For this review, use the dimensioned drawing (mm, ordinates from the lowest corner) and the shaded views. A direction names the side the tool comes from. Coordinates: 2 decimals unless noted, no trailing zeros. Loops run counter-clockwise (first coordinate to the right, second up) from the corner with the lowest first, then second, coordinate; pieces in that order, holes last. Notation, with made-up numbers: (55, 47) - (86, 47) arc R33 cw to (86, 84) - close; hole circle Ø2 at (10.25, 88). An arc over 180 degrees is marked (long way). One line per item, written item: value. Start each with the question number.
1. For the marked faces 5, 6, 7 and 8, list the 3-axis set-ups (+Z, -Z, +X, -X, +Y, -Y) from which the entire face can be reached by the end or side of a thin tool; tool diameter is ignored.
2. To check wall thickness, follow line 1 (Z direction, x = 27.5, y = 14.75); line 2 (Y direction, x = 1.75, z = 13). State the ranges of each line that lie inside material, in increasing order.
3. Insertion check: P1, Ø2.5, axis at y = 2, z = 18.5, coming from the -X side; P2, Ø2, axis at x = 22.5, y = 22, coming from the -Z side; P3, Ø2.5, axis at x = 16.5, z = 2.5, coming from the +Y side. Each pin has a flat end and moves straight along its axis. Give the tip position at first contact, or say it passes through.
4. Mouldability with a two-part tool opening along Z and no side actions: class the marked faces 1, 2, 3 and 4 as +Z half, -Z half, draft (parallel to the pull), parting line (faces both ways), or undercut.
5. We need section C-C, the plane x = 18. Give the boundary of the cut face in (y, z), then the cut area to 3 significant figures.
6. We need section B-B, the plane y = 28. Give the boundary of the cut face in (x, z), then the cut area to 3 significant figures.
7. We need section D-D, the plane x = 26.75. Give the boundary of the cut face in (y, z), then the cut area to 3 significant figures.
8. We need section A-A, the plane z = 23. Give the boundary of the cut face in (x, y).
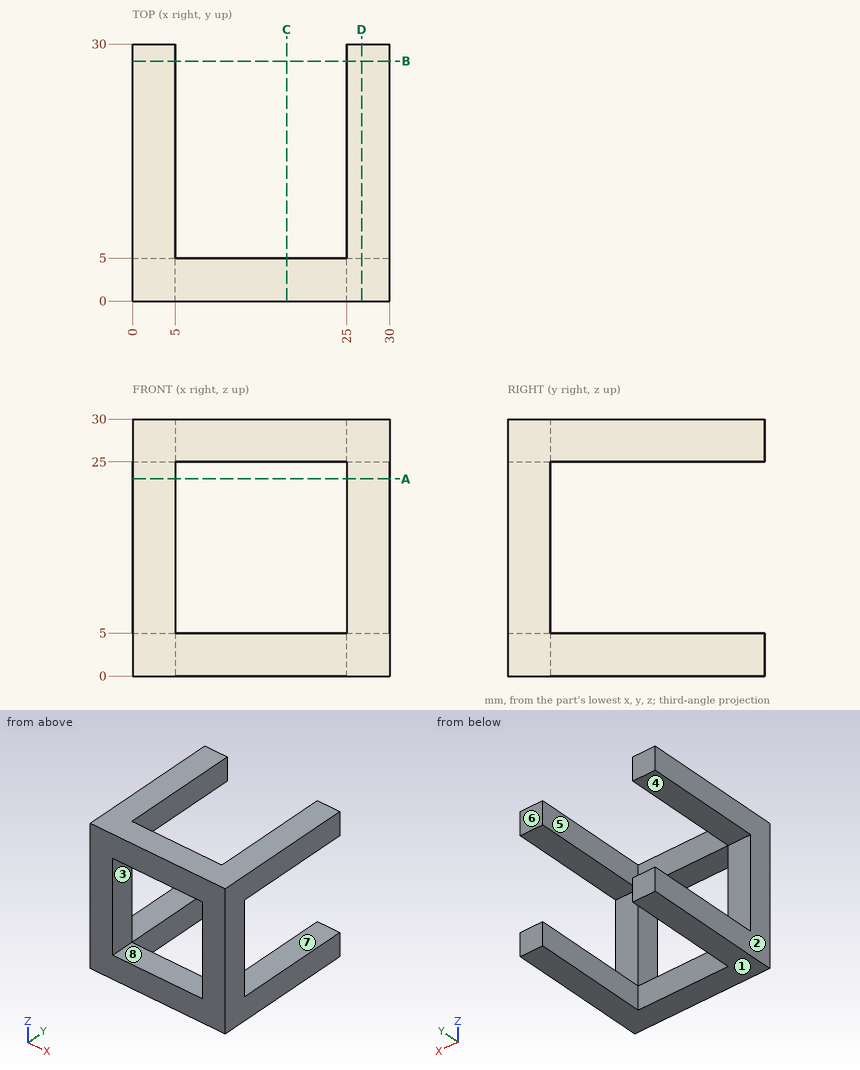
Findings below:
1. face 5: +Z, -Z, +Y
1. face 6: +Z, -Z, +X, -X, +Y
1. face 7: +X, -X, +Y
1. face 8: +Y, -Y
2. line 1: 0 to 5, 25 to 30
2. line 2: 0 to 5
3. P1: x = 0
3. P2: through
3. P3: y = 5
4. face 1: -Z half
4. face 2: draft
4. face 3: undercut
4. face 4: undercut
5. outline: (0, 0) - (5, 0) - (5, 5) - (0, 5) - close; (0, 25) - (5, 25) - (5, 30) - (0, 30) - close
5. area: 50.0 mm2
6. outline: (0, 0) - (5, 0) - (5, 5) - (0, 5) - close; (0, 25) - (5, 25) - (5, 30) - (0, 30) - close; (25, 0) - (30, 0) - (30, 5) - (25, 5) - close; (25, 25) - (30, 25) - (30, 30) - (25, 30) - close
6. area: 100 mm2
7. outline: (0, 0) - (30, 0) - (30, 5) - (5, 5) - (5, 25) - (30, 25) - (30, 30) - (0, 30) - close
7. area: 400 mm2
8. outline: (0, 0) - (5, 0) - (5, 5) - (0, 5) - close; (25, 0) - (30, 0) - (30, 5) - (25, 5) - close
